Can you work these out from the model? Positions are in its coordinate system, mm. Face numbers are marked on the shaded views. A direction names the side the tool comes from. Round coordinates to 2 decimals unless told otherwise and drop trailing zeros. Loops run counter-clockwise (first coordinate to the right, second up) from the corner with the lowest first, then second, coordinate; pieces in that order, holes last.
from build123d import *

# Parameters (mm, degrees)
F0_W     = 50.8
F0_H     = 50.8
F1_DEPTH = 38.1
F2_SIZE  = 5.08


with BuildPart() as f1:
    # F0 (on Front) → F1 (new body)
    with BuildSketch(Plane.XZ):
        with BuildLine():
            Line((-14.8284427494, 76.4413994114), (-116.4284427494, 76.4413994114))
            ThreePointArc((-116.4284427494, 76.4413994114), (-125.4086988705, 72.7216555324), (-129.1284427494, 63.7413994114))
            Line((-129.1284427494, 63.7413994114), (-129.1284427494, -37.8586005886))
            ThreePointArc((-129.1284427494, -37.8586005886), (-125.4086988705, -46.8388567097), (-116.4284427494, -50.5586005886))
            Line((-116.4284427494, -50.5586005886), (-14.8284427494, -50.5586005886))
            ThreePointArc((-14.8284427494, -50.5586005886), (-2.1284427494, -37.8586005886), (10.5715572506, -50.5586005886))
            Line((10.5715572506, -50.5586005886), (112.1715572506, -50.5586005886))
            ThreePointArc((112.1715572506, -50.5586005886), (121.1518133717, -46.8388567097), (124.8715572506, -37.8586005886))
            Line((124.8715572506, -37.8586005886), (124.8715572506, 63.7413994114))
            ThreePointArc((124.8715572506, 63.7413994114), (121.1518133717, 72.7216555324), (112.1715572506, 76.4413994114))
            Line((112.1715572506, 76.4413994114), (10.5715572506, 76.4413994114))
            ThreePointArc((10.5715572506, 76.4413994114), (-2.1284427494, 63.7413994114), (-14.8284427494, 76.4413994114))
        make_face()
        with Locations((-2.1284427494, 12.9413994114)):
            Rectangle(F0_W, F0_H, mode=Mode.SUBTRACT)
    extrude(amount=F1_DEPTH)

    # F2
    f2_edges = [f1.edges().sort_by_distance(p)[0] for p in [
        (23.271557, -19.05, 38.341399),
        (23.271557, -19.05, -12.458601),
        (23.271557, 0, 12.941399),
        (23.271557, -38.1, 12.941399),
        (-27.528443, -19.05, 38.341399),
        (-2.128443, 0, 38.341399),
        (-2.128443, -38.1, 38.341399),
        (-27.528443, 0, 12.941399),
        (-27.528443, -38.1, 12.941399),
        (-2.128443, 0, -12.458601),
        (-2.128443, -38.1, -12.458601),
    ]]
    chamfer(f2_edges, length=F2_SIZE)


solid = f1.part
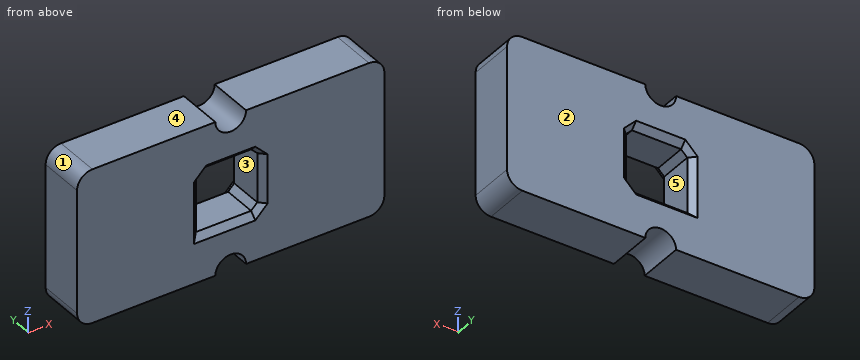
(1) For the marked faces 4 and 5, which set-ups out of +Z, -Z, +X, -X, +Y, -Y let a thin tool reach every point of the face, with its end or its side?
Worked answers:
face 4: +Z, +X, -X, +Y, -Y
face 5: +Y, -Y
(2) If we mould it in two halves opening along Z, with no side actions, what happens to the marked faces 1, 2 and 3? For each: released by +Z, released by -Z, zero draft, split by the parting line, or undercut.
Worked answers:
face 1: released by +Z
face 2: zero draft
face 3: undercut
(3) If we section it at B-B, the plane y = -8.5: List the corners of the cut face in (x, z) for me.
Worked answers:
outline: (-129.13, -37.86) arc R12.7 ccw to (-116.43, -50.56) - (-14.83, -50.56) arc R12.7 cw to (10.57, -50.56) - (112.17, -50.56) arc R12.7 ccw to (124.87, -37.86) - (124.87, 63.74) arc R12.7 ccw to (112.17, 76.44) - (10.57, 76.44) arc R12.7 cw to (-14.83, 76.44) - (-116.43, 76.44) arc R12.7 ccw to (-129.13, 63.74) - close; hole (-27.53, -12.46) - (18.19, -12.46) - (23.27, -7.38) - (23.27, 33.26) - (18.19, 38.34) - (-22.45, 38.34) - (-27.53, 33.26) - close
(4) If we section it at A-A, the plane z = -2: List the corners of the cut face in (x, y) for me, then the cut area to 3 significant figures.
Worked answers:
outline: (-129.13, -38.1) - (-32.61, -38.1) - (-27.53, -33.02) - (-27.53, -5.08) - (-32.61, 0) - (-129.13, 0) - close; (23.27, -33.02) - (28.35, -38.1) - (124.87, -38.1) - (124.87, 0) - (28.35, 0) - (23.27, -5.08) - close
area: 7,690 mm2
(5) If we section it at C-C, the plane z = 69: List the corners of the cut face in (x, y) for me, then the cut area to 3 significant figures.
Worked answers:
outline: (-127.99, -38.1) - (-12.42, -38.1) - (-12.42, 0) - (-127.99, 0) - close; (8.16, -38.1) - (123.73, -38.1) - (123.73, 0) - (8.16, 0) - close
area: 8,810 mm2
(6) If I drill on line 1 (X direction, y = -27, z = 21); line 2 (X direction, y = -17, z = 37); line 3 (Z direction, x = 114, y = -4), over which ranges is the centre line in solid material (lowest first)?
Worked answers:
line 1: x = -129.13 to -27.53, 23.27 to 124.87
line 2: x = -129.13 to -23.79, 19.53 to 124.87
line 3: z = -50.43 to 76.31
